from build123d import *

# Parameters (mm, degrees)
CUT_EXTRUDE1_DEPTH = 201


with BuildPart() as part:
    # Sketch1 → Revolve1 (revolve)
    with BuildSketch(Plane.XY):
        Polygon((-100, 6.35), (100, 6.35), (100, 16.51), (93.65, 16.51), (93.65, 12.7), (-93.65, 12.7), (-93.65, 16.51), (-100, 16.51), align=None)
    revolve(axis=Axis((0, 0, 0), (1, 0, 0)))

    # Sketch2 → Cut-Extrude1 (cut, through all)
    with BuildSketch(Plane(origin=(100, 0, 0), x_dir=(0, 0, -1), z_dir=(1, 0, 0))):
        Polygon((3.666174209, 6.35), (-3.666174209, 6.35), (-7.332348419, 0), (-3.666174209, -6.35), (3.666174209, -6.35), (7.332348419, 0), align=None)
    extrude(amount=-CUT_EXTRUDE1_DEPTH, mode=Mode.SUBTRACT)


solid = part.part
Verification items for the finished model (mm, model axes). A direction names the side the tool comes from. Coordinates: 2 decimals unless noted, no trailing zeros. Order: outer loops, then holes, each group sorted by start corner. A loop starts at its lowest first (then second) coordinate and runs counter-clockwise, first axis right, second up. Notation, with made-up numbers: M -25.75,1.5 L 19.25,1.5 A21 cw 19.25,31.5 Z; hole C -29,79 d7. An arc over 180 degrees is marked long. One line per item, written item: value. Start each with the question number.
Item 1: Scan lines: probe 1 along X at (y, z) = (8.5, 12.5); probe 2 along Y at (x, z) = (26.5, -1); probe 3 along Y at (x, z) = (-83, 4). Record each from-to range of solid material in increasing order.
Item 2: Access from +Z, -Z, +X, -X, +Y, -Y to the whole of each face (thin tool, end or side, straight path). Record for faces 1 (the flat face through (1.4, -3.131, 5.525)), 2 (the flat face through (-93.65, -8.5, -9.7)), 3 (the flat face through (100, -7, 0)).
Item 3: Sectioned sample at B-B (z = 0). Enter the section's corners in (x, y), then the cut area to 3 significant figures.
Item 4: Mould release check, pull along Y, two halves, no side actions. Record for faces 4 (the flat face through (93.65, 8.5, -9.7)), 5 (the flat face through (1, -6.35, 0)), 6 (the cylindrical face through (-1.31, -2.75, -12.4)): released by +Y, released by -Y, zero draft, split by the parting line, or undercut.
Item 5: Sectioned sample at C-C (y = -9.5). Enter the section's corners in (x, z), then the cut area to 3 significant figures.
Item 6: Sectioned sample at A-A (x = -67). Enter the section's corners in (y, z).
Item 7: Gauge pin test, flat ends, axial feed: pin 1 (1 mm diameter, centred on x = -49.5, y = 8, fed in from +Z); pin 2 (3 mm diameter, centred on y = 1, z = 4.5, fed in from -X); pin 3 (3.5 mm diameter, centred on x = 17.5, z = -1, fed in from -Y); pin 4 (1.5 mm diameter, centred on x = -43.5, y = -7.5, fed in from +Z). Record the tip position at first contact, or that the pin passes through.
Item 8: Sectioned sample at D-D (z = 10). Enter the section's corners in (x, y).
Conclusion:
1. probe 1: x = -100 to -93.65, 93.65 to 100
1. probe 2: y = -12.66 to -6.35, 6.35 to 12.66
1. probe 3: y = -12.05 to -5.77, 5.77 to 12.05
2. face 1: +X, -X
2. face 2: none
2. face 3: +Z, -Z, +X, +Y, -Y
3. outline: M -100,-16.51 L -93.65,-16.51 L -93.65,-12.7 L 93.65,-12.7 L 93.65,-16.51 L 100,-16.51 L 100,-6.35 L -100,-6.35 Z; M -100,6.35 L 100,6.35 L 100,16.51 L 93.65,16.51 L 93.65,12.7 L -93.65,12.7 L -93.65,16.51 L -100,16.51 Z
3. area: 2,640 mm^2
4. face 4: zero draft
4. face 5: undercut
4. face 6: split by the parting line
5. outline: M -100,-13.5 L -93.65,-13.5 L -93.65,-8.43 L 93.65,-8.43 L 93.65,-13.5 L 100,-13.5 L 100,13.5 L 93.65,13.5 L 93.65,8.43 L -93.65,8.43 L -93.65,13.5 L -100,13.5 Z
5. area: 3,500 mm^2
6. outline: C 0,0 d25.4; hole M -6.35,-3.67 L 0,-7.33 L 6.35,-3.67 L 6.35,3.67 L 0,7.33 L -6.35,3.67 Z
7. pin 1: stops at z = 10.25
7. pin 2: passes through
7. pin 3: stops at y = -12.7
7. pin 4: stops at z = 10.76
8. outline: M -100,-13.14 L -93.65,-13.14 L -93.65,-7.83 L 93.65,-7.83 L 93.65,-13.14 L 100,-13.14 L 100,13.14 L 93.65,13.14 L 93.65,7.83 L -93.65,7.83 L -93.65,13.14 L -100,13.14 Z
